Work out the finished part from the listing and answer in its coordinate system (mm). Coordinates: 2 decimals unless noted, no trailing zeros. Order: outer loops, then holes, each group sorted by start corner. A loop starts at its lowest first (then second) coordinate and runs counter-clockwise, first axis right, second up. Notation, with made-up numbers: M -15.5,-23.75 L -6.5,-23.75 A20 cw -6.5,13.25 Z; hole C -17,33 d2. An arc over 180 degrees is marked long. Use a Markdown table: item, result.
from build123d import *

# Parameters (mm, degrees)
SKETCH_1_W          = 300
SKETCH_1_H          = 300
EXTRUDE_1_DEPTH     = 10
SKETCH_2_R          = 20
CUT_EXTRUDE_1_DEPTH = 213.367605816
SKETCH_3_W          = 300
SKETCH_3_H          = 10
EXTRUDE_2_DEPTH     = 25


with BuildPart() as part:
    # 草图1 → 凸台-拉伸1 (new body)
    with BuildSketch(Plane.XY):
        Rectangle(SKETCH_1_W, SKETCH_1_H)
    extrude(amount=EXTRUDE_1_DEPTH)

    # 草图2 → 切除-拉伸1 (cut, through all)
    with BuildSketch(Plane.XY.offset(10)):
        with Locations((-70, -70)):
            Circle(SKETCH_2_R)
        with Locations((71.421356237, -20)):
            Circle(SKETCH_2_R)
    extrude(amount=-CUT_EXTRUDE_1_DEPTH, mode=Mode.SUBTRACT)

    # 草图3 → 凸台-拉伸2 (add)
    with BuildSketch(Plane.XZ.offset(150)):
        with Locations((0, 5)):
            Rectangle(SKETCH_3_W, SKETCH_3_H)
    extrude(amount=EXTRUDE_2_DEPTH)


solid = part.part
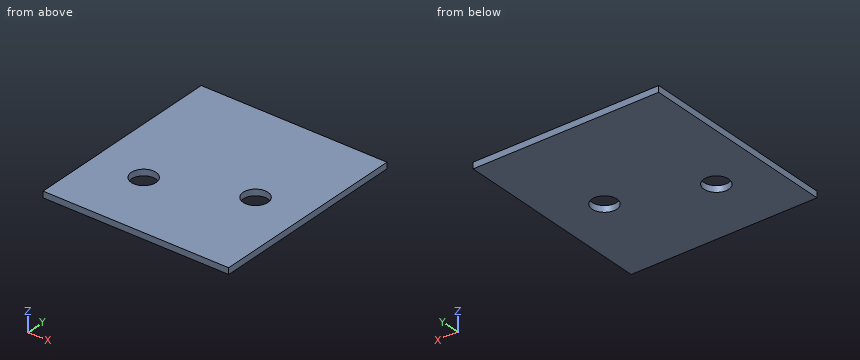
(1) A cutting plane is placed at C-C (z = 4.5). Determine the outline of the cut face in (x, y), then the cut area to 3 significant figures.
Conclusion:
| item | result |
|---|---|
| outline | M -150,-175 L 150,-175 L 150,150 L -150,150 Z; hole C -70,-70 d40; hole C 71.42,-20 d40 |
| area | 95,000 mm2 |
(2) A cutting plane is placed at A-A (x = -70). Determine the outline of the cut face in (y, z).
Conclusion:
| item | result |
|---|---|
| outline | M -175,0 L -90,0 L -90,10 L -175,10 Z; M -50,0 L 150,0 L 150,10 L -50,10 Z |
(3) A cutting plane is placed at B-B (y = -70). Determine the outline of the cut face in (x, z).
Conclusion:
| item | result |
|---|---|
| outline | M -150,0 L -90,0 L -90,10 L -150,10 Z; M -50,0 L 150,0 L 150,10 L -50,10 Z |
(4) Straight lines are drawn through the part: L1, parallel to Y at x = -70, z = 6.75; L2, parallel to Y at x = -85, z = 4.5; L3, parallel to X at y = -38.5, z = 1. For each, find the intervals that lie inside material, in ascending order.
Conclusion:
| item | result |
|---|---|
| L1 | -175 to -90, -50 to 150 |
| L2 | -175 to -83.23, -56.77 to 150 |
| L3 | -150 to 63.82, 79.02 to 150 |
